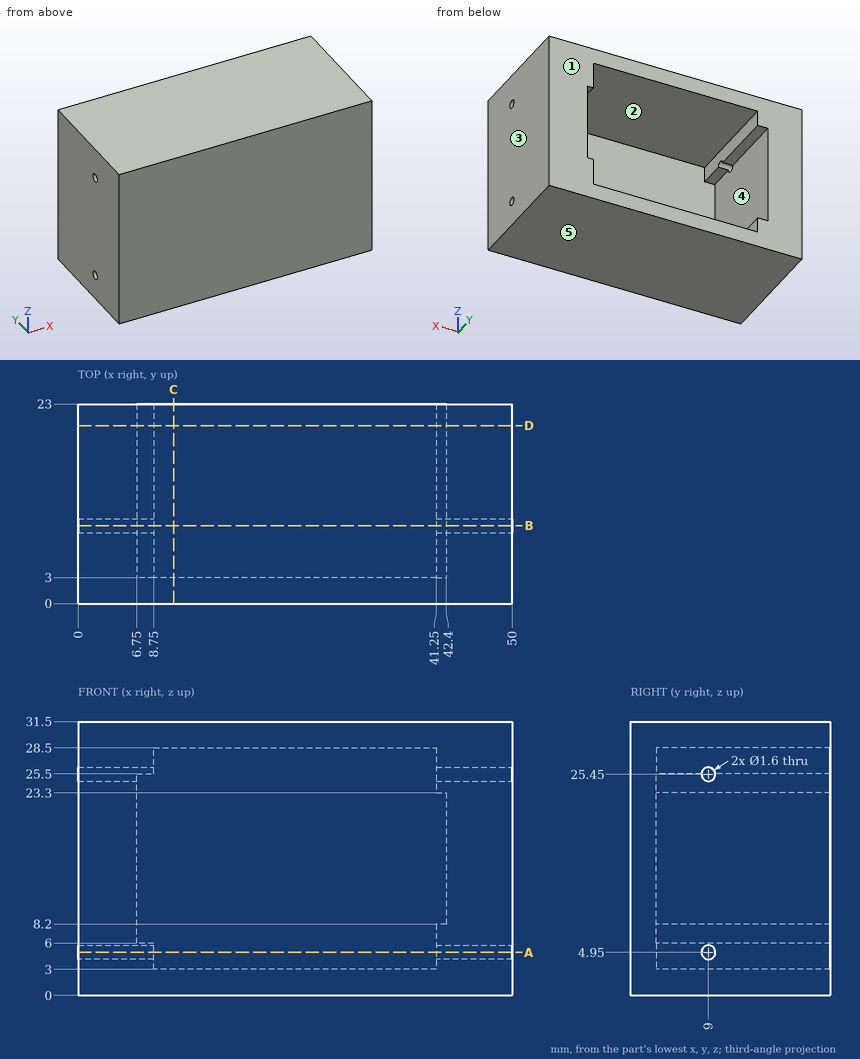
Could you check a few things on this drawing? It's one solid part, dimensions in mm from its lowest x, y, z. A direction names the side the tool comes from. Coordinates: 2 decimals unless noted, no trailing zeros. Order: outer loops, then holes, each group sorted by start corner. A loop starts at its lowest first (then second) coordinate and runs counter-clockwise, first axis right, second up.
1) Imagine slicing it at A-A on z = 4.95. List the corners of the cut face in (x, y) for me, and give its area (3 significant figures).
2) Imagine slicing it at C-C on x = 11. List the corners of the cut face in (y, z) for me.
3) Which directions (+Z, -Z, +X, -X, +Y, -Y) give clear straight access to the entire face, cutting with the end or side of a thin tool? Please do the marked faces 4 and 5.
4) Will these pins go through, and if not, where does the flat tip stop? pin 1 (2 mm diameter, centred on x = 30.5, z = 9, fed in from +Y); pin 2 (1 mm diameter, centred on y = 9, z = 4.95, fed in from -X).
5) I need wall thicknesses on line 1 (Y direction, x = 3.5, z = 4.95); line 2 (Z direction, x = 29.5, y = 11.5); line 3 (X direction, y = 6.5, z = 21.5). Which ranges of each line are inside material? Lowest first, please.
6) Imagine slicing it at D-D on y = 20.5. List the corners of the cut face in (x, z) for me.
7) We'd pull the mould along X, two halves only. Please class the marked faces 1, 2 and 3: +X half, -X half, draft (parallel to the pull), parting line (faces both ways), or undercut.
8) Imagine slicing it at B-B on y = 9. State how many separate pieces and enclosed holes the cut face has, and give its area (3 significant figures).
Response values:
1. outline: (0, 0) - (50, 0) - (50, 8.2) - (41.25, 8.2) - (41.25, 3) - (8.75, 3) - (8.75, 8.2) - (0, 8.2) - close; (0, 9.8) - (8.75, 9.8) - (8.75, 23) - (0, 23) - close; (41.25, 9.8) - (50, 9.8) - (50, 23) - (41.25, 23) - close
1. area: 472 mm2
2. outline: (0, 0) - (23, 0) - (23, 3) - (3, 3) - (3, 28.5) - (23, 28.5) - (23, 31.5) - (0, 31.5) - close
3. face 4: +Y
3. face 5: -Z, +X, -X, +Y, -Y
4. pin 1: stops at y = 3
4. pin 2: passes through
5. line 1: y = 0 to 8.2, 9.8 to 23
5. line 2: z = 0 to 3, 28.5 to 31.5
5. line 3: x = 0 to 6.75, 42.4 to 50
6. outline: (0, 0) - (50, 0) - (50, 31.5) - (0, 31.5) - close; hole (6.75, 6) - (8.75, 6) - (8.75, 3) - (41.25, 3) - (41.25, 8.2) - (42.4, 8.2) - (42.4, 23.3) - (41.25, 23.3) - (41.25, 28.5) - (8.75, 28.5) - (8.75, 25.5) - (6.75, 25.5) - close
7. face 1: draft
7. face 2: undercut
7. face 3: +X half
8. separate pieces: 4
8. enclosed holes: 0
8. area: 636 mm2
